The model under review builds one solid part; all positions refer to its coordinate system, in mm. Face numbers are marked on the shaded views. A direction names the side the tool comes from. Coordinates: 2 decimals unless noted, no trailing zeros. Write each loop counter-clockwise with the first axis right and the second up, starting at its lowest first coordinate (ties: lowest second). Pieces come first, ordered by that corner, then holes. Notation, with made-up numbers: M 51.5,-29 L 80.5,-29 A27 cw 80.5,2 Z; hole C -36.75,3.25 d4. An arc over 180 degrees is marked long. Answer as CSV lines item,"result". Start each with the question number.
from build123d import *

# Parameters (mm, degrees)
EXTRUDE_THIN1_DEPTH = 10
SKETCH2_W           = 7
SKETCH2_H           = 7
BOSS_EXTRUDE1_DEPTH = 2
FILLET1_R           = 1
CUT_EXTRUDE1_REACH  = 45.1
SKETCH3_W           = 10
SKETCH3_H           = 28.8
SKETCH4_W           = 9
SKETCH4_H           = 28.8
BOSS_EXTRUDE2_DEPTH = 2
BOSS_EXTRUDE3_DEPTH = 6.4
SKETCH6_R           = 1.065
CUT_EXTRUDE2_DEPTH  = 44.1


with BuildPart() as part:
    # Sketch1 → Extrude-Thin1 (new body)
    with BuildSketch(Plane.XY):
        Polygon((-2, -36.8), (-2, -5), (-2, 2), (41.1, 2), (41.1, -36.8), (34.1, -36.8), align=None)
        Polygon((0, -34.8), (0, -5), (0, 0), (39.1, 0), (39.1, -34.8), (34.1, -34.8), align=None, mode=Mode.SUBTRACT)
    extrude(amount=-EXTRUDE_THIN1_DEPTH)

    # Sketch2 → Boss-Extrude1 (add)
    with BuildSketch(Plane.XY):
        with Locations((3.5, -3.5)):
            Rectangle(SKETCH2_W, SKETCH2_H)
        with Locations((35.6, -3.5)):
            Rectangle(SKETCH2_W, SKETCH2_H)
        with Locations((35.6, -31.3)):
            Rectangle(SKETCH2_W, SKETCH2_H)
        with Locations((3.5, -31.3)):
            Rectangle(SKETCH2_W, SKETCH2_H)
    extrude(amount=-BOSS_EXTRUDE1_DEPTH)

    # Fillet1
    fillet1_edges = [part.edges().sort_by_distance(p)[0] for p in [
        (7, -7, -1),
        (32.1, -7, -1),
        (32.1, -27.8, -1),
        (7, -27.8, -1),
    ]]
    fillet(fillet1_edges, radius=FILLET1_R)


with BuildPart() as body_2:
    # Mirror1: mirrored copy
    add(part.part.mirror(Plane(origin=(39.1, 0, -10), x_dir=(0, 0, 1), z_dir=(1, 0, 0))))

    # Sketch3 → Cut-Extrude1 (cut, up to next)
    with BuildSketch(Plane.ZY.offset(-37.1), mode=Mode.PRIVATE) as cut_extrude1_sk1:
        with Locations((-5, -16.4)):
            Rectangle(SKETCH3_W, SKETCH3_H)
    cut_extrude1_tool1 = extrude(cut_extrude1_sk1.sketch, amount=-CUT_EXTRUDE1_REACH, mode=Mode.PRIVATE) & body_2.part
    add(cut_extrude1_tool1.solids().sort_by_distance((37.1, -16.4, -5))[0], mode=Mode.SUBTRACT)

    # Sketch4 → Boss-Extrude2 (add)
    with BuildSketch(Plane.XY):
        with Locations((41.6, -16.4)):
            Rectangle(SKETCH4_W, SKETCH4_H)
    extrude(amount=-BOSS_EXTRUDE2_DEPTH)

    # Sketch5 → Boss-Extrude3 (add)
    with BuildSketch(Plane.XY):
        Polygon((71.2, -34.8), (71.2, -36.8), (80.2, -36.8), (80.2, -27.8), (78.2, -27.8), (78.2, -34.8), align=None)
    boss_extrude3 = extrude(amount=BOSS_EXTRUDE3_DEPTH)

    # Mirror2: Boss-Extrude3 across plane
    add(boss_extrude3.mirror(Plane.ZX.offset(-17.4)))

    # Mirror3: Boss-Extrude3 across plane
    add(boss_extrude3.mirror(Plane(origin=(58.65, 0, 0), x_dir=(0, 0, 1), z_dir=(1, 0, 0))))

    # Sketch6 → Cut-Extrude2 (cut, through all)
    with BuildSketch(Plane(origin=(80.2, 0, 0), x_dir=(0, 0, -1), z_dir=(1, 0, 0))):
        with Locations((-3.4, -32.8)):
            Circle(SKETCH6_R)
    cut_extrude2 = extrude(amount=-CUT_EXTRUDE2_DEPTH, mode=Mode.SUBTRACT)

    # Mirror4: Cut-Extrude2 across plane
    add(cut_extrude2.mirror(Plane.ZX.offset(-17.4)), mode=Mode.SUBTRACT)


solid = body_2.part
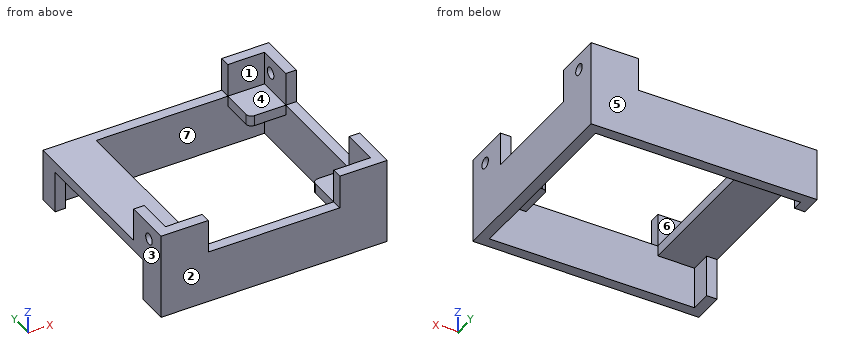
1) Tool access review of the marked faces 4, 5, 6 and 7: name each direction out of +Z, -Z, +X, -X, +Y, -Y from which nothing blocks a thin tool from reaching the whole face with its end or side.
2) To check wall thickness, follow line 1 (Y direction, x = 38.15, z = 3.4) (3 decimals); line 2 (Y direction, x = 79.15, z = 3.4) (3 decimals); line 3 (Y direction, x = 72, z = -2.5). State the ranges of each line that lie inside material, in increasing order. Write a range as [from, to].
3) Mouldability with a two-part tool opening along Y and no side actions: class the marked faces 1, 2 and 3 as +Y half, -Y half, draft (parallel to the pull), parting line (faces both ways), or undercut.
4) Take a section at B-B on z = 3.4. Give the number of separate pieces and of enclosed holes in the cut face, and give its area (3 significant figures).
5) Clearance check with flat-ended pins moving along their axes: pin 1 Ø5 at (y, z) = (-5, 3.5) entering from -X; pin 2 Ø3.5 at (y, z) = (-32.8, 3.4) entering from +X; pin 3 Ø2 at (x, y) = (75.5, -33) entering from +Z; pin 4 Ø8 at (x, y) = (42.5, -25.5) entering from -Z. State where each tip first meets the part, or that it passes through.
6) Take a section at D-D on z = -1. Give the boundary of the cut face in (x, y), and give its area (3 significant figures).
7) Take a section at A-A on x = 64.5. Give the boundary of the cut face in (y, z).
8) Take a section at C-C on y = -32.8. Give the boundary of the cut face in (x, z) (3 decimals).
Results:
1,face 4,"+Z, -X"
1,face 5,"+Z, -Z, +X, -X, +Y"
1,face 6,"+Z, +Y"
1,face 7,"-Z"
2,line 1,"y = [-36.8, -33.865], [-31.735, -27.8]"
2,line 2,"y = [-36.8, -33.865], [-31.735, -27.8], [-7, -3.065], [-0.935, 2]"
2,line 3,"y = [-36.8, -34.8], [0, 2]"
3,face 1,"undercut"
3,face 2,"-Y half"
3,face 3,"draft"
4,separate pieces,"6"
4,enclosed holes,"0"
4,area,"83.2 mm²"
5,pin 1,"stops at x = 78.2"
5,pin 2,"stops at x = 80.2"
5,pin 3,"stops at z = 0"
5,pin 4,"stops at z = -2"
6,outline,"M 37.1,-36.8 L 80.2,-36.8 L 80.2,2 L 37.1,2 Z; hole M 46.1,-34.8 L 71.2,-34.8 L 71.2,-28.8 A1 cw 72.2,-27.8 L 78.2,-27.8 L 78.2,-7 L 72.2,-7 A1 cw 71.2,-6 L 71.2,0 L 46.1,0 Z"
6,area,"653 mm²"
7,outline,"M -36.8,-10 L -34.8,-10 L -34.8,0 L -36.8,0 Z; M 0,-10 L 2,-10 L 2,0 L 0,0 Z"
8,outline,"M 37.1,-10 L 39.1,-10 L 39.1,-2 L 46.1,-2 L 46.1,0 L 39.1,0 L 39.1,2.335 L 37.1,2.335 Z; M 37.1,4.465 L 39.1,4.465 L 39.1,6.4 L 37.1,6.4 Z; M 71.2,-2 L 78.2,-2 L 78.2,-10 L 80.2,-10 L 80.2,2.335 L 78.2,2.335 L 78.2,0 L 71.2,0 Z; M 78.2,4.465 L 80.2,4.465 L 80.2,6.4 L 78.2,6.4 Z"
